Design review of the part built by this model. Coordinates are the model's own, in mm. Coordinates: 2 decimals unless noted, no trailing zeros. Write each loop counter-clockwise with the first axis right and the second up, starting at its lowest first coordinate (ties: lowest second). Pieces come first, ordered by that corner, then holes.
Q1. Take a section at B-B (z = 9.5). Give the boundary of the cut face in (x, y), and give its area (3 significant figures).
Q2. For probe 1 along Y at (x, z) = (0, 7); probe 2 along X at (y, z) = (-2, 3); probe 3 along Y at (x, z) = (-7.25, 2.5), list the stretches that pass through material, from the lowest coordinate up.
Q3. Mouldability with a two-part tool opening along Y and no side actions: class faces 1 (the conical face through (6.248, 10.76, 9.844)), 2 (the conical face through (-6.248, -10.76, 0.256)), 3 (the cylindrical face through (1.73, -7.81, 4.98)) as pulls with the +Y half, pulls with the -Y half, needs draft (parallel to the pull), parting line crosses it, or undercut.
Q4. Take a section at A-A (z = 2). Give the boundary of the cut face in (x, y), and give its area (3 significant figures).
Q5. Insertion check: pin 1 (5 mm diameter, centred on y = -4.5, z = 9, fed in from -X); pin 2 (13 mm diameter, centred on x = 0, y = 0, fed in from +Z); pin 3 (1 mm diameter, centred on y = -3.5, z = 3.5, fed in from -X); pin 4 (5 mm diameter, centred on x = -5.5, y = 7, fed in from -Z). Each pin has a flat end and moves straight along its axis. Give the tip position at first contact, or say it passes through.
```python
from build123d import *

# Parameters (mm, degrees)
BOSS_EXTRUDE1_DEPTH = 10.1
SKETCH2_OUTSIDE_W   = 113.28
SKETCH2_OUTSIDE_H   = 109.568
SKETCH2_OUTSIDE_R   = 12
CUT_EXTRUDE1_DEPTH  = 21.928688444
CUT_EXTRUDE1_DRAFT  = -60
SKETCH8_R           = 8
CUT_EXTRUDE4_DEPTH  = 21.928688444
SKETCH9_OUTSIDE_W   = 113.28
SKETCH9_OUTSIDE_H   = 109.568
SKETCH9_OUTSIDE_R   = 12
CUT_EXTRUDE6_DEPTH  = 21.928688444
CUT_EXTRUDE6_DRAFT  = 60


with BuildPart() as part:
    # Sketch1 → Boss-Extrude1 (new body)
    with BuildSketch(Plane.XY):
        Polygon((13.856406461, 0), (6.92820323, 12), (-6.92820323, 12), (-13.856406461, 0), (-6.92820323, -12), (6.92820323, -12), align=None)
    extrude(amount=BOSS_EXTRUDE1_DEPTH)


with BuildPart() as cut_extrude1_tool:
    # Sketch2 outside → Cut-Extrude1 (with draft: the straight prism first)
    with BuildSketch(Plane.XY.offset(10.1)):
        Rectangle(SKETCH2_OUTSIDE_W, SKETCH2_OUTSIDE_H)
        Circle(SKETCH2_OUTSIDE_R, mode=Mode.SUBTRACT)
    extrude(amount=-CUT_EXTRUDE1_DEPTH)
    # Cut-Extrude1: the draft: its side faces are tilted about the plane it starts from
    cut_extrude1_sides = [cut_extrude1_tool.faces().sort_by_distance(p)[0] for p in [
        (0, -54.784, -0.864344222),
        (56.64, 0, -0.864344222),
        (0, 54.784, -0.864344222),
        (-56.64, 0, -0.864344222),
        (-12, 0, -0.864344222),
    ]]
    draft(cut_extrude1_sides, Plane.XY.offset(10.1), CUT_EXTRUDE1_DRAFT)


with BuildPart() as part_1:
    add(part.part)

    # Cut-Extrude1: cut by cut_extrude1_tool
    add(cut_extrude1_tool.part, mode=Mode.SUBTRACT)

    # Sketch8 → Cut-Extrude4 (cut, through all)
    with BuildSketch(Plane(origin=(0, 0, 0), x_dir=(-1, 0, 0), z_dir=(0, 0, -1))):
        Circle(SKETCH8_R)
    extrude(amount=-CUT_EXTRUDE4_DEPTH, mode=Mode.SUBTRACT)


with BuildPart() as cut_extrude6_tool:
    # Sketch9 outside → Cut-Extrude6 (with draft: the straight prism first)
    with BuildSketch(Plane.XY):
        Rectangle(SKETCH9_OUTSIDE_W, SKETCH9_OUTSIDE_H)
        Circle(SKETCH9_OUTSIDE_R, mode=Mode.SUBTRACT)
    extrude(amount=CUT_EXTRUDE6_DEPTH)
    # Cut-Extrude6: the draft: its side faces are tilted about the plane it starts from
    cut_extrude6_sides = [cut_extrude6_tool.faces().sort_by_distance(p)[0] for p in [
        (0, -54.784, 10.964344222),
        (56.64, 0, 10.964344222),
        (0, 54.784, 10.964344222),
        (-56.64, 0, 10.964344222),
        (-12, 0, 10.964344222),
    ]]
    draft(cut_extrude6_sides, Plane.XY, CUT_EXTRUDE6_DRAFT)


with BuildPart() as part_2:
    add(part_1.part)

    # Cut-Extrude6: cut by cut_extrude6_tool
    add(cut_extrude6_tool.part, mode=Mode.SUBTRACT)


solid = part_2.part
```
Response:
1. outline: (-12.94, -1.58) - (-7.84, -10.42) arc R13.04 ccw to (-5.1, -12) - (5.1, -12) arc R13.04 ccw to (7.84, -10.42) - (12.94, -1.58) arc R13.04 ccw to (12.94, 1.58) - (7.84, 10.42) arc R13.04 ccw to (5.1, 12) - (-5.1, 12) arc R13.04 ccw to (-7.84, 10.42) - (-12.94, 1.58) arc R13.04 ccw to start; hole circle Ø16 at (0, 0)
1. area: 290 mm2
2. probe 1: y = -12 to -8, 8 to 12
2. probe 2: x = -12.7 to -7.75, 7.75 to 12.7
2. probe 3: y = -11.44 to -3.38, 3.38 to 11.44
3. face 1: pulls with the +Y half
3. face 2: pulls with the -Y half
3. face 3: undercut
4. outline: (-13.86, 0) - (-6.93, -12) - (6.93, -12) - (13.86, 0) - (6.93, 12) - (-6.93, 12) - close; hole circle Ø16 at (0, 0)
4. area: 298 mm2
5. pin 1: stops at x = -12.7
5. pin 2: passes through
5. pin 3: stops at x = -12.12
5. pin 4: stops at z = 0
